```python
from build123d import *

# Parameters (mm, degrees)
F_1_8_0_125_DIAMETER_HOLE1_D = 3.175
CIRPATTERN1_COUNT            = 8


with BuildPart() as part:
    # Sketch1 → Revolve1 (revolve)
    with BuildSketch(Plane.XY):
        with BuildLine():
            Line((3.592102448, 17.562102448), (13.570307345, 7.583897552))
            ThreePointArc((13.570307345, 7.583897552), (15.218377957, 6.482691975), (17.162409794, 6.096))
            ThreePointArc((17.162409794, 6.096), (17.493946322, 6.117730052), (17.819810168, 6.182548401))
            Line((17.819810168, 6.182548401), (20.340629853, 6.858))
            Line((20.340629853, 6.858), (20.340629853, 13.208))
            Line((20.340629853, 13.208), (16.926461018, 13.208))
            Line((16.926461018, 13.208), (3.175, 26.959461018))
            Line((3.175, 26.959461018), (3.175, 38.1))
            Line((3.175, 38.1), (0, 38.1))
            Line((0, 38.1), (0, 19.05))
            ThreePointArc((0, 19.05), (1.944031836, 18.663308025), (3.592102448, 17.562102448))
        make_face()
    revolve(axis=Axis((0, 0, 0), (1, 0, 0)))

    # 1_8 _0.125_ Diameter Hole1 (through all)
    with Locations(Plane(origin=(3.175, 0, 0), x_dir=(0, 0, -1), z_dir=(1, 0, 0))):
        with Locations((0, 31.75)):
            f_1_8_0_125_diameter_hole1 = Hole(F_1_8_0_125_DIAMETER_HOLE1_D / 2)

    # CirPattern1: 1_8 _0.125_ Diameter Hole1 ×8 about axis
    cirpattern1_axis = Axis((0, 0, 0), (1, 0, 0))
    for i in range(1, CIRPATTERN1_COUNT):
        add(f_1_8_0_125_diameter_hole1.rotate(cirpattern1_axis, i * 360 / CIRPATTERN1_COUNT), mode=Mode.SUBTRACT)


solid = part.part
```
Read the model definition and answer for the solid it produces. Units are mm, in the model's axes. Give positions to 0.01 mm unless a question says otherwise; leave off trailing zeros. Loops run counter-clockwise (first coordinate to the right, second up) from the corner with the lowest first, then second, coordinate; pieces in that order, holes last.
Item 1: The part is cut by section A-A (z = 31.75). Write down the section's boundary in (x, y) (1 decimal), and give its area (3 significant figures).
Item 2: The part is cut by section C-C (z = 0). Give the number of separate pieces and of enclosed holes in the cut face, and give its area (3 significant figures).
Item 3: Each of these flat-tipped pins is pushed along its axis until it touches: pin 1 Ø3 at (y, z) = (31.75, 0) entering from +X; pin 2 Ø1 at (x, z) = (17, 4) entering from -Y; pin 3 Ø10 at (x, y) = (13, 9) entering from -Z; pin 4 Ø3 at (x, y) = (6, -8.5) entering from +Z. Where does it stop, or does it pass through?
Item 4: The mould has two halves that part along Z. Classify faces 1 (the cylindrical face through (1.57, -0.85, 33.09)), 2 (the flat face through (3.175, -8, 26)), 3 (the cylindrical face through (18.61, 12.2, -5.06)): released by +Z, released by -Z, zero draft, split by the parting line, or undercut.
Item 5: The part is cut by section D-D (x = 6). Write down the section's boundary in (y, z).
Item 6: Find the intervals of material crossed by line 1 along Z through (x, y) = (1, 0); line 2 along Z through (x, y) = (1.9, 0); line 3 along X through (y, z) = (-35, 6) (3 decimals), in increasing order.
Taken from the geometry:
1. outline: (0, -21.1) - (3.2, -21.1) - (3.2, -1.6) - (0, -1.6) - close; (0, 1.6) - (3.2, 1.6) - (3.2, 21.1) - (0, 21.1) - close
1. area: 124 mm2
2. separate pieces: 4
2. enclosed holes: 0
2. area: 392 mm2
3. pin 1: passes through
3. pin 2: stops at y = -13.06
3. pin 3: stops at z = -20.58
3. pin 4: stops at z = 24.26
4. face 1: undercut
4. face 2: zero draft
4. face 3: split by the parting line
5. outline: circle Ø48.27 at (0, 0); hole circle Ø30.31 at (0, 0)
6. line 1: z = -38.1 to -33.34, -30.16 to -18.95, 18.95 to 30.16, 33.34 to 38.1
6. line 2: z = -38.1 to -33.34, -30.16 to -18.68, 18.68 to 30.16, 33.34 to 38.1
6. line 3: x = 0 to 3.175
